from build123d import *

# Parameters (mm, degrees)
F0_W      = 14.6957188845
F0_H      = 34.1013113993
F0_W_2    = 45.72
F0_H_2    = 34.1122
F0_H_3    = 9.7971446812
F0_W_3    = 45.7200031853
F1_DEPTH  = 182.372
F2_T      = -2.54
F3_W      = 5.08
F3_H      = 2.54
F4_DEPTH  = 25.4
F5_W      = 5.08
F5_H      = 5.08
F6_DEPTH  = 25.4
F7_W      = 5.08
F7_H      = 2.54
F8_DEPTH  = 25.4
F9_W      = 5.08
F9_H      = 2.54
F10_DEPTH = 10.3632


with BuildPart() as f1:
    # F0 (on Front) → F1 (new body)
    with BuildSketch(Plane.XZ):
        with Locations((-68.5800015926, 39.0107723406)):
            Rectangle(F0_W, F0_H)
        with Locations((-38.3721421504, 4.9040166409)):
            Rectangle(F0_W_2, F0_H_2)
        with Locations((-68.5800015926, 4.9040166409)):
            Rectangle(F0_W, F0_H_2)
        with Locations((-68.5800015926, -29.2081833591)):
            Rectangle(F0_W, F0_H_2)
        with Locations((-68.5800015926, -51.1628556997)):
            Rectangle(F0_W, F0_H_3)
        with Locations((-38.3721421504, -29.2081833591)):
            Rectangle(F0_W_2, F0_H_2)
        with Locations((-38.3721421504, -51.1628556997)):
            Rectangle(F0_W_2, F0_H_3)
        with Locations((7.3478594422, -51.1628556997)):
            Rectangle(F0_W_3, F0_H_3)
        with Locations((53.0678610349, -51.1628556997)):
            Rectangle(F0_W_2, F0_H_3)
        with Locations((7.3478594422, -29.2081833591)):
            Rectangle(F0_W_3, F0_H_2)
    extrude(amount=F1_DEPTH)

    # F2
    f2_openings = [f1.faces().sort_by_distance(p)[0] for p in [
        (0, -91.186, -56.061428),
    ]]
    offset(amount=F2_T, openings=f2_openings, kind=Kind.INTERSECTION)

    # F3 (on face) → F4 (cut)
    with BuildSketch(Plane.YZ.offset(30.2078610349)):
        with Locations((-157.226, -27.9381833591)):
            Rectangle(F3_W, F3_H)
        with Locations((-157.226, -30.4781833591)):
            Rectangle(F3_W, F3_H)
        with Locations((-124.206, -30.4781833591)):
            Rectangle(F3_W, F3_H)
        with Locations((-124.206, -27.9381833591)):
            Rectangle(F3_W, F3_H)
        with Locations((-91.186, -30.4781833591)):
            Rectangle(F3_W, F3_H)
        with Locations((-91.186, -27.9381833591)):
            Rectangle(F3_W, F3_H)
        with Locations((-58.166, -30.4781833591)):
            Rectangle(F3_W, F3_H)
        with Locations((-58.166, -27.9381833591)):
            Rectangle(F3_W, F3_H)
        with Locations((-25.146, -27.9381833591)):
            Rectangle(F3_W, F3_H)
        with Locations((-25.146, -30.4781833591)):
            Rectangle(F3_W, F3_H)
    extrude(amount=-F4_DEPTH, mode=Mode.SUBTRACT)

    # F5 (on face) → F6 (cut)
    with BuildSketch(Plane.XZ.offset(182.372)):
        with Locations((-68.675249815, -50.2550639212)):
            Rectangle(F5_W, F5_H)
    extrude(amount=-F6_DEPTH, mode=Mode.SUBTRACT)

    # F7 (on face) → F8 (cut)
    with BuildSketch(Plane.YZ.offset(-15.5121421504)):
        with Locations((-157.3796552205, 5.9143330357)):
            Rectangle(F7_W, F7_H)
        with Locations((-157.3796552205, 3.3743330357)):
            Rectangle(F7_W, F7_H)
        with Locations((-124.3596552205, 5.9143330357)):
            Rectangle(F7_W, F7_H)
        with Locations((-124.3596552205, 3.3743330357)):
            Rectangle(F7_W, F7_H)
        with Locations((-91.3396552205, 5.9143330357)):
            Rectangle(F7_W, F7_H)
        with Locations((-91.3396552205, 3.3743330357)):
            Rectangle(F7_W, F7_H)
        with Locations((-58.3196552205, 5.9143330357)):
            Rectangle(F7_W, F7_H)
        with Locations((-58.3196552205, 3.3743330357)):
            Rectangle(F7_W, F7_H)
        with Locations((-25.2996552205, 5.9143330357)):
            Rectangle(F7_W, F7_H)
        with Locations((-25.2996552205, 3.3743330357)):
            Rectangle(F7_W, F7_H)
    extrude(amount=-F8_DEPTH, mode=Mode.SUBTRACT)

    # F9 (on face) → F10 (cut)
    with BuildSketch(Plane.YZ.offset(-61.2321421504)):
        with Locations((-157.3776137614, 41.7377093029)):
            Rectangle(F9_W, F9_H)
        with Locations((-157.3776137614, 39.1977093029)):
            Rectangle(F9_W, F9_H)
        with Locations((-124.3576137614, 41.7377093029)):
            Rectangle(F9_W, F9_H)
        with Locations((-124.3576137614, 39.1977093029)):
            Rectangle(F9_W, F9_H)
        with Locations((-91.3376137614, 41.7377093029)):
            Rectangle(F9_W, F9_H)
        with Locations((-91.3376137614, 39.1977093029)):
            Rectangle(F9_W, F9_H)
        with Locations((-58.3176137614, 41.7377093029)):
            Rectangle(F9_W, F9_H)
        with Locations((-58.3176137614, 39.1977093029)):
            Rectangle(F9_W, F9_H)
        with Locations((-25.2976137614, 41.7377093029)):
            Rectangle(F9_W, F9_H)
        with Locations((-25.2976137614, 39.1977093029)):
            Rectangle(F9_W, F9_H)
    extrude(amount=-F10_DEPTH, mode=Mode.SUBTRACT)


solid = f1.part
Input: part model. Units: mm. Frame: model coordinates. A direction names the side the tool comes from. Give positions to 0.01 mm unless a question says otherwise; leave off trailing zeros. Write each loop counter-clockwise with the first axis right and the second up, starting at its lowest first coordinate (ties: lowest second). Pieces come first, ordered by that corner, then holes.
Q1. Pull-direction query (X, two-part tool) for faces 4 (the face through (30.208, -90, -33)), 5 (the face through (-35, 0, -24)), 6 (the face through (-34, -179.832, -25)), 7 (the face through (-69, -90, 53.521)); classes: pulls with the +X half, pulls with the -X half, needs draft (parallel to the pull), parting line crosses it, or undercut.
Q2. Section D-D, the plane z = -36. Output: boundary loops of the cut face in (x, y), plus the area to 3 significant figures.
Q3. First-contact query: P1, Ø3, axis at x = -62.5, y = -157.5, coming from the -Z side; P2, Ø3, axis at x = -45, y = -122.5, coming from the +Z side; P3, Ø1.5, axis at y = -117, z = 38.5, coming from the +X side. Flat tips, straight axial feed; report the tip coordinate or a pass-through.
Q4. Set-up query: faces 1 (the face through (-15.512, -90, 8)), 2 (the face through (-34, -2.54, -25)), 3 (the face through (75.928, -90, -51)). Return all of +Z, -Z, +X, -X, +Y, -Y with unobstructed straight access to the full face (end or side cutting, diameter ignored); none if empty.
Q5. Section A-A, the plane z = 26. Output: boundary loops of the cut face in (x, y), plus the area to 3 significant figures.
Q6. Material intervals for probe 1 along X at (y, z) = (-156.5, -37); probe 2 along Y at (x, z) = (-18, -35.5); probe 3 along X at (y, z) = (-82.5, 33.5), sorted ascending.
Q7. Section C-C, the plane y = -110. Output: boundary loops of the cut face in (x, z).
Q8. Section B-B, the plane x = 6. Output: boundary loops of the cut face in (y, z), plus the area to 3 significant figures.
Filled in:
1. face 4: pulls with the +X half
1. face 5: needs draft
1. face 6: undercut
1. face 7: undercut
2. outline: (-75.93, -182.37) - (30.21, -182.37) - (30.21, 0) - (-75.93, 0) - close; hole (-73.39, -179.83) - (27.67, -179.83) - (27.67, -2.54) - (-73.39, -2.54) - close
2. area: 1,440 mm2
3. P1: stops at z = 19.42
3. P2: stops at z = 21.96
3. P3: stops at x = -61.23
4. face 1: +Z, +X, +Y, -Y
4. face 2: -Z
4. face 3: +Z, -Z, +X, +Y, -Y
5. outline: (-75.93, -182.37) - (-61.23, -182.37) - (-61.23, 0) - (-75.93, 0) - close; hole (-73.39, -179.83) - (-63.77, -179.83) - (-63.77, -2.54) - (-73.39, -2.54) - close
5. area: 975 mm2
6. probe 1: x = -75.93 to -73.39, 27.67 to 30.21
6. probe 2: y = -182.37 to -179.83, -2.54 to 0
6. probe 3: x = -75.93 to -73.39, -63.77 to -61.23
7. outline: (-75.93, -56.06) - (-73.39, -56.06) - (-73.39, 53.52) - (-63.77, 53.52) - (-63.77, 19.42) - (-18.05, 19.42) - (-18.05, -14.69) - (27.67, -14.69) - (27.67, -48.8) - (73.39, -48.8) - (73.39, -56.06) - (75.93, -56.06) - (75.93, -46.26) - (30.21, -46.26) - (30.21, -12.15) - (-15.51, -12.15) - (-15.51, 21.96) - (-61.23, 21.96) - (-61.23, 56.06) - (-75.93, 56.06) - close
8. outline: (-182.37, -56.06) - (-179.83, -56.06) - (-179.83, -14.69) - (-2.54, -14.69) - (-2.54, -56.06) - (0, -56.06) - (0, -12.15) - (-182.37, -12.15) - close
8. area: 673 mm2
